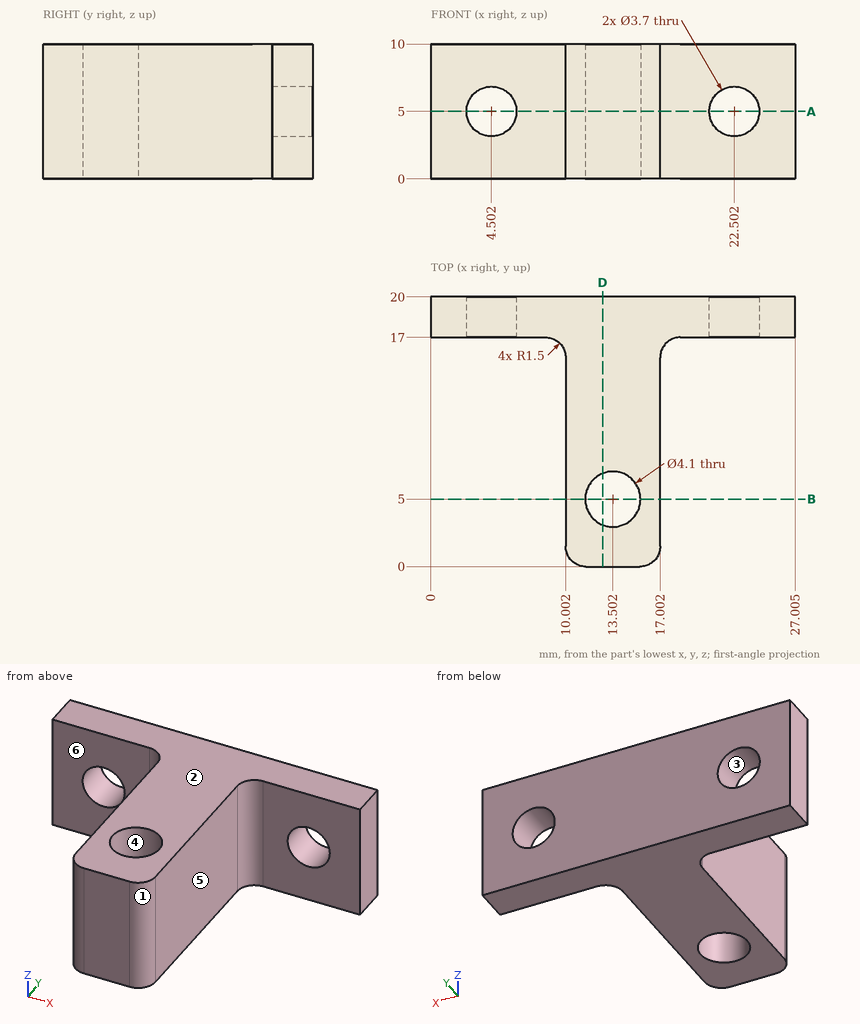
Here's the drawing with two shaded views (mm, measured from the low corner). I have some questions. A direction names the side the tool comes from. Give positions to 0.01 mm unless a question says otherwise; leave off trailing zeros. Write each loop counter-clockwise with the first axis right and the second up, starting at its lowest first coordinate (ties: lowest second). Pieces come first, ordered by that corner, then holes. Notation, with made-up numbers: (-1.5, -26.5) - (40.5, -26.5) arc R15 cw to (40.5, -12.5) - close; hole circle Ø11 at (-6.75, 58.5). An arc over 180 degrees is marked (long way). One line per item, written item: value. Start each with the question number.
Item 1: Imagine slicing it at B-B, the plane y = 5. List the corners of the cut face in (x, z) for me.
Item 2: I'm going to push flat-ended pins straight in: pin 1 (1.5 mm diameter, centred on y = 7.5, z = 7.5, fed in from +X); pin 2 (6 mm diameter, centred on y = 14.5, z = 5.5, fed in from -X); pin 3 (1 mm diameter, centred on y = 6, z = 5.5, fed in from -X); pin 4 (4.5 mm diameter, centred on x = 24.5, z = 6, fed in from -Y). Where does each tip first touch, or does it pass through?
Item 3: Which directions (+Z, -Z, +X, -X, +Y, -Y) give clear straight access to the entire face, cutting with the end or side of a thin tool? Please do the marked faces 4, 5 and 6.
Item 4: Imagine slicing it at D-D, the plane x = 12.75. List the corners of the cut face in (y, z) for me.
Item 5: If we mould it in two halves opening along Z, with no side actions, what happens to the marked faces 1, 2 and 3? For each: +Z half, -Z half, draft (parallel to the pull), parting line (faces both ways), or undercut.
Item 6: Imagine slicing it at A-A, the plane z = 5. Give the number of separate pieces and of enclosed holes in the cut face, and give its area (3 significant figures).
Item 7: Please list where these lines run through material, in increasing order: line 1 (X direction, y = 17.85, z = 5) (1 decimal); line 2 (Y direction, x = 22, z = 2); line 3 (X direction, y = 13.5, z = 9). Write a range as from..to.
Geometry says:
1. outline: (10, 0) - (11.45, 0) - (11.45, 10) - (10, 10) - close; (15.55, 0) - (17, 0) - (17, 10) - (15.55, 10) - close
2. pin 1: x = 17
2. pin 2: x = 0
2. pin 3: x = 10
2. pin 4: y = 17
3. face 4: +Z, -Z
3. face 5: +Z, -Z, +X, -Y
3. face 6: +Z, -Z, -X, -Y
4. outline: (0, 0) - (3.09, 0) - (3.09, 10) - (0, 10) - close; (6.91, 0) - (20, 0) - (20, 10) - (6.91, 10) - close
5. face 1: draft
5. face 2: +Z half
5. face 3: undercut
6. separate pieces: 3
6. enclosed holes: 1
6. area: 165 mm^2
7. line 1: 0..2.7, 6.4..20.7, 24.4..27
7. line 2: 17..20
7. line 3: 10..17
